Geometry check sheet. Reference: drawing and pictorial views, mm from the part's lowest x, y, z. A direction names the side the tool comes from. Round coordinates to 2 decimals unless told otherwise and drop trailing zeros. Order: outer loops, then holes, each group sorted by start corner. A loop starts at its lowest first (then second) coordinate and runs counter-clockwise, first axis right, second up.
Q1. Scan lines: probe 1 along Z at (x, y) = (11.75, 8); probe 2 along Y at (x, z) = (22.5, 3.75); probe 3 along Z at (x, y) = (22, 22.5). Record each from-to range of solid material in increasing order.
Q2. Cross-section at D-D on x = 4. Record the cut outline in (y, z), then the cut area to 3 significant figures.
Q3. Mould release check, pull along Z, two halves, no side actions. Record for the marked faces 4, 5, 6 and 7: +Z half, -Z half, draft (parallel to the pull), parting line (faces both ways), or undercut.
Q4. Cross-section at C-C on z = 10. Record the cut outline in (x, y).
Q5. Depth check by flat-ended pin: P1, Ø3, axis at x = 18, y = 20, coming from the -Z side; P2, Ø8, axis at x = 19.5, z = 8.5, coming from the -Y side; P3, Ø6, axis at x = 22, z = 10, coming from the -Y side; P4, Ø5, axis at y = 6.5, z = 10, coming from the +X side. Enter the tip coordinate at first touch or a pass-through.
Q6. Cross-section at B-B on y = 8. Record the cut outline in (x, z).
Q7. Cross-section at A-A on x = 22. Record the cut outline in (y, z).
Q8. Set-up check for the marked faces 1, 2 and 3: record each of +Z, -Z, +X, -X, +Y, -Y from which the full face is reachable in a straight line by a thin tool's end or side.
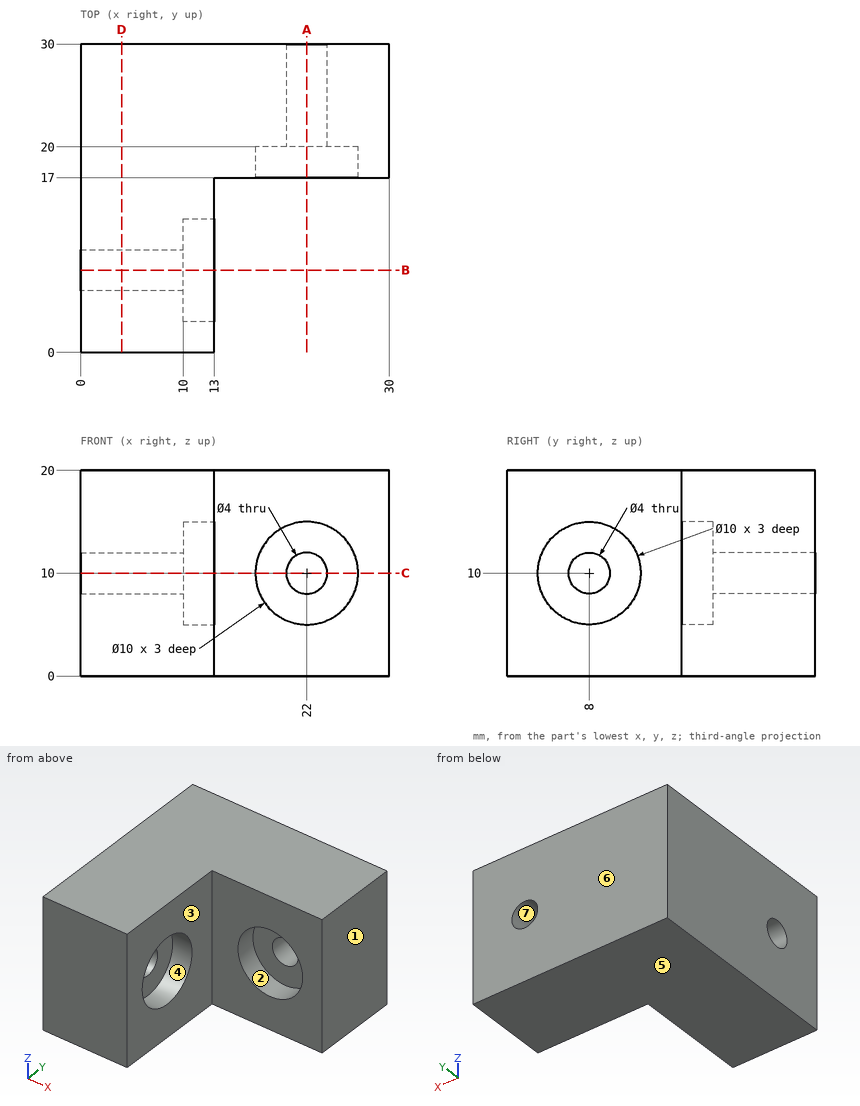
Results found:
1. probe 1: z = 0 to 5, 15 to 20
1. probe 2: y = 17 to 30
1. probe 3: z = 0 to 8, 12 to 20
2. outline: (0, 0) - (30, 0) - (30, 20) - (0, 20) - close; hole circle Ø4 at (8, 10)
2. area: 587 mm2
3. face 4: undercut
3. face 5: -Z half
3. face 6: draft
3. face 7: undercut
4. outline: (0, 0) - (13, 0) - (13, 3) - (10, 3) - (10, 6) - (0, 6) - close; (0, 10) - (10, 10) - (10, 13) - (13, 13) - (13, 17) - (17, 17) - (17, 20) - (20, 20) - (20, 30) - (0, 30) - close; (24, 20) - (27, 20) - (27, 17) - (30, 17) - (30, 30) - (24, 30) - close
5. P1: stops at z = 0
5. P2: stops at y = 17
5. P3: stops at y = 20
5. P4: stops at x = 10
6. outline: (0, 0) - (13, 0) - (13, 5) - (10, 5) - (10, 8) - (0, 8) - close; (0, 12) - (10, 12) - (10, 15) - (13, 15) - (13, 20) - (0, 20) - close
7. outline: (17, 0) - (30, 0) - (30, 8) - (20, 8) - (20, 5) - (17, 5) - close; (17, 15) - (20, 15) - (20, 12) - (30, 12) - (30, 20) - (17, 20) - close
8. face 1: +Z, -Z, +X, +Y, -Y
8. face 2: -Y
8. face 3: +Z, -Z, +X, -Y
